The figure shows three views and two pictorial views of one solid part (mm, origin at its lowest corner). Answer the questions. A direction names the side the tool comes from. Coordinates: 2 decimals unless noted, no trailing zeros. Order: outer loops, then holes, each group sorted by start corner. A loop starts at its lowest first (then second) coordinate and runs counter-clockwise, first axis right, second up. Notation, with made-up numbers: (89, 82.25) -> (114, 82.25) arc R32 cw to (114, 116.25) -> close; hole circle Ø10 at (73.25, 48.5). An arc over 180 degrees is marked (long way). Return JSON: item names as keys, results as strings.
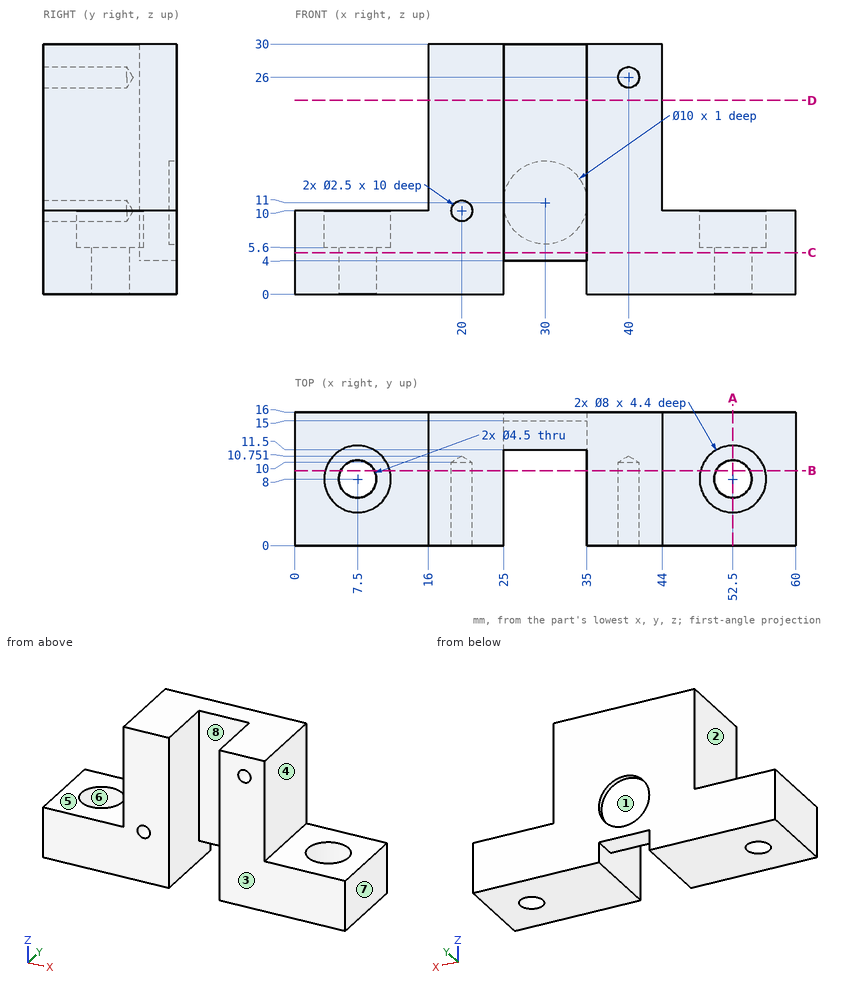
1. The part is cut by section B-B on y = 9. Give the number of separate pieces and of enclosed holes in the cut face, and give its area (3 significant figures).
Answer block:
{"separate pieces": "4", "enclosed holes": "2", "area": "737 mm2"}
2. For the marked faces 4, 5, 6, 7 and 8, determine the directions among +Z, -Z, +X, -X, +Y, -Y from which every point of the face is accessible in a straight line to the end or side of a thin tool.
Answer block:
{"face 4": "+Z, +X, +Y, -Y", "face 5": "+Z, -X, +Y, -Y", "face 6": "+Z", "face 7": "+Z, -Z, +X, +Y, -Y", "face 8": "+Z, -Z, -Y"}
3. Each of these flat-tipped pins is pushed along its axis until it touches: pin 1 Ø6 at (y, z) = (14, 3) entering from -X; pin 2 Ø8 at (y, z) = (8.5, 22.5) entering from -X; pin 3 Ø5 at (x, y) = (7.5, 8) entering from +Z; pin 4 Ø4 at (x, y) = (9.5, 11) entering from +Z. Where does it stop, or does it pass through?
Answer block:
{"pin 1": "stops at x = 0", "pin 2": "stops at x = 16", "pin 3": "stops at z = 5.6", "pin 4": "stops at z = 10"}
4. The part is cut by section A-A on x = 52.5. Give the vertices of the cut face in (y, z).
Answer block:
{"outline": "(0, 0) -> (5.75, 0) -> (5.75, 5.6) -> (4, 5.6) -> (4, 10) -> (0, 10) -> close; (10.25, 0) -> (16, 0) -> (16, 10) -> (12, 10) -> (12, 5.6) -> (10.25, 5.6) -> close"}
5. The part is cut by section D-D on z = 23.25. Give the vertices of the cut face in (x, y), and give its area (3 significant figures).
Answer block:
{"outline": "(16, 0) -> (25, 0) -> (25, 11.5) -> (35, 11.5) -> (35, 0) -> (44, 0) -> (44, 16) -> (16, 16) -> close", "area": "333 mm2"}
6. Determine the mould class of the marked faces 1, 2 and 3 for opening direction X: pulls with the +X half, pulls with the -X half, needs draft (parallel to the pull), parting line crosses it, or undercut.
Answer block:
{"face 1": "undercut", "face 2": "pulls with the -X half", "face 3": "needs draft"}
7. Consider line 1 (X direction, y = 8, z = 3.55); line 2 (X direction, y = 5.5, z = 26); line 3 (X direction, y = 6, z = 13). Determine where each line is inside the solid, lowest interval first. Write a range as from..to.
Answer block:
{"line 1": "x = 0..5.25, 9.75..25, 35..50.25, 54.75..60", "line 2": "x = 16..25, 35..38.75, 41.25..44", "line 3": "x = 16..25, 35..44"}
8. The part is cut by section C-C on z = 5. Give the vertices of the cut face in (x, y).
Answer block:
{"outline": "(0, 0) -> (25, 0) -> (25, 11.5) -> (35, 11.5) -> (35, 0) -> (60, 0) -> (60, 16) -> (0, 16) -> close; hole circle Ø4.5 at (7.5, 8); hole circle Ø4.5 at (52.5, 8)"}
